from build123d import *

# Parameters (mm, degrees)
F0_W     = 14.444813
F0_H     = 75.975604
F1_DEPTH = 34.479829
F2_R     = 5.454239
F3_DEPTH = 1.041855
F4_SIZE  = 4.572


with BuildPart() as f1:
    # F0 (on Front) → F1 (new body)
    with BuildSketch(Plane.XZ):
        with Locations((7.222406, 37.987802)):
            Rectangle(F0_W, F0_H)
    extrude(amount=-F1_DEPTH)

    # F2 (on face) → F3 (join)
    with BuildSketch(Plane.XZ):
        with Locations((7.329378, 65.214992)):
            Circle(F2_R)
    extrude(amount=F3_DEPTH)

    # F4
    f4_edges = [f1.edges().sort_by_distance(p)[0] for p in [
        (7.222407, 0, 75.975604),
        (7.222407, 0, 0),
    ]]
    chamfer(f4_edges, length=F4_SIZE)


solid = f1.part
For this review, take the finished solid that the model builds, in its own axes (mm). A direction names the side the tool comes from. Give positions to 0.01 mm unless a question says otherwise; leave off trailing zeros. Loops run counter-clockwise (first coordinate to the right, second up) from the corner with the lowest first, then second, coordinate; pieces in that order, holes last. Notation, with made-up numbers: (-30.75, 25.25) -> (-8.75, 25.25) arc R9 cw to (-8.75, 30.25) -> close; hole circle Ø1 at (-9.75, 37). An arc over 180 degrees is marked (long way). One line per question, with ' | ' between items.
1) We need section B-B (z = 11). Write out the cut boundary in (x, y), plus the area to 3 significant figures.
Resolved:
outline: (0, 0) -> (14.44, 0) -> (14.44, 34.48) -> (0, 34.48) -> close | area: 498 mm2
2) Insertion check: pin 1 Ø1 at (x, y) = (6.5, 3.5) entering from -Z; pin 2 Ø8 at (x, z) = (3.5, 16.5) entering from -Y. Each pin has a flat end and moves straight along its axis. Give the tip position at first contact, or say it passes through.
Resolved:
pin 1: stops at z = 0.57 | pin 2: stops at y = 0
3) We need section C-C (y = 2). Write out the cut boundary in (x, z).
Resolved:
outline: (0, 2.57) -> (14.44, 2.57) -> (14.44, 73.4) -> (0, 73.4) -> close
4) We need section D-D (x = 13.5). Write out the cut boundary in (y, z), plus the area to 3 significant figures.
Resolved:
outline: (0, 4.57) -> (4.57, 0) -> (34.48, 0) -> (34.48, 75.98) -> (4.57, 75.98) -> (0, 71.4) -> close | area: 2,600 mm2
5) To check wall thickness, follow probe 1 along Y at (x, z) = (7, 43); probe 2 along Z at (x, y) = (13, 2.5); probe 3 along Y at (x, z) = (13.5, 4). State the ranges of each line that lie inside material, in increasing order.
Resolved:
probe 1: y = 0 to 34.48 | probe 2: z = 2.07 to 73.9 | probe 3: y = 0.57 to 34.48
6) We need section A-A (x = 3.5). Write out the cut boundary in (y, z).
Resolved:
outline: (-1.04, 61.33) -> (0, 61.33) -> (0, 4.57) -> (4.57, 0) -> (34.48, 0) -> (34.48, 75.98) -> (4.57, 75.98) -> (0, 71.4) -> (0, 69.1) -> (-1.04, 69.1) -> close
7) For faces 1 (the flat face through (7, 19, 0)), 2 (the cylindrical face through (6.1, -0.5, 59.9)), list the 3-axis set-ups (+Z, -Z, +X, -X, +Y, -Y) from which the entire face can be reached by the end or side of a thin tool; tool diameter is ignored.
Resolved:
face 1: -Z, +X, -X, +Y, -Y | face 2: -Y
